Autodesk Inventor part; units mm, degrees
ref_plane "YZ Plane" through (0, 0, 0) normal (1, 0, 0) x (0, 1, 0)
ref_plane "XZ Plane" through (0, 0, 0) normal (0, 1, 0) x (-1, 0, 0)
ref_plane "XY Plane" through (0, 0, 0) normal (0, 0, 1) x (1, 0, 0)
sketch "Sketch1" plane through (0, 0, 0) normal (0, 0, 1) x (1, 0, 0)
  line L0 (-34.925, 22.225) -> (34.925, 22.225)
  line L1 (34.925, 22.225) -> (34.925, -22.225)
  line L2 (34.925, -22.225) -> (-34.925, -22.225)
  line L3 (-34.925, -22.225) -> (-34.925, 22.225)
  point P0 (0, 0)
  dimension "d0" = 69.85
  dimension "d1" = 44.45
  dimension "d2" = 34.925
  dimension "d3" = 22.225
extrude "Extrusion1" add sketch "Sketch1" along normal mid plane 4.7625
sketch "Sketch2" plane through (0, 0, 2.3813) normal (0, 0, 1) x (1, 0, 0)
  line L0 (-34.925, -22.225) -> (-34.925, 22.225)
  line L1 (34.925, -22.225) -> (-34.925, -22.225)
  point P0 (-19.05, 3.175)
  point P1 (19.05, 3.175)
  dimension "d6" = 25.4
  dimension "d7" = 15.875
  dimension "d8" = 38.1
hole "Hole1" at (-19.05, 3.175, 2.3813) at (19.05, 3.175, 2.3813) direction (0, 0, -1) diameter 6.7564 depth 19.05 tip angle 118 countersink diameter 12.8778 countersink angle 82
properties part number "Jaw_Plate" material "Steel, High Strength Low Alloy"
Verification items for the finished model (mm, model axes). Coordinates: 2 decimals unless noted, no trailing zeros. Order: outer loops, then holes, each group sorted by start corner. A loop starts at its lowest first (then second) coordinate and runs counter-clockwise, first axis right, second up. Notation, with made-up numbers: M 37.25,-26.5 L 87.25,-26.5 A17 cw 87.25,-20.5 Z; hole C 59,83.5 d11. An arc over 180 degrees is marked long. Write each question's results on one line, items separated by ' | '.
1) Section check A-A on x = 19.05. Record the cut outline in (y, z) (3 decimals).
Solved:
outline: M -22.225,-2.381 L -0.203,-2.381 L -0.203,-1.14 L -3.264,2.381 L -22.225,2.381 Z; M 6.553,-2.381 L 22.225,-2.381 L 22.225,2.381 L 9.614,2.381 L 6.553,-1.14 Z
2) Scan lines: line 1 along Y through (x, z) = (19.05, -1.85) (3 decimals); line 2 along X through (y, z) = (5, -2.05) (3 decimals); line 3 along X through (y, z) = (0.5, 0.1) (1 decimal). Record each from-to range of solid material in increasing order. Write a range as [from, to].
Solved:
line 1: y = [-22.225, -0.203], [6.553, 22.225] | line 2: x = [-34.925, -21.893], [-16.207, 16.207], [21.893, 34.925] | line 3: x = [-34.9, -22.6], [-15.5, 15.5], [22.6, 34.9]
3) Section check C-C on y = 5.5. Give the number of separate pieces and of enclosed holes in the cut face, plus the area to 3 significant figures.
Solved:
separate pieces: 3 | enclosed holes: 0 | area: 260 mm²
4) Section check B-B on z = 0.9. Record the cut outline in (x, y) (3 decimals), plus the area to 3 significant figures.
Solved:
outline: M -34.925,-22.225 L 34.925,-22.225 L 34.925,22.225 L -34.925,22.225 Z; hole C -19.05,3.175 d10.302; hole C 19.05,3.175 d10.302 | area: 2,940 mm²
5) Release check for a two-part mould opening along X. For faces 1 (the face through (16.2, 1.36, -1.77)), 2 (the face through (0, 0, -2.381)), 3 (the face through (-34.925, 0, 0)) record: pulls with the +X half, pulls with the -X half, needs draft (parallel to the pull), parting line crosses it, or undercut.
Solved:
face 1: undercut | face 2: needs draft | face 3: pulls with the -X half
6) Gauge pin test, flat ends, axial feed: pin 1 Ø9 at (x, y) = (19.05, 3.175) entering from -Z; pin 2 Ø8 at (x, y) = (-19.05, 3.175) entering from +Z. Record the tip position at first contact, or that the pin passes through.
Solved:
pin 1: stops at z = -2.38 | pin 2: stops at z = -0.42
